```python
from build123d import *

# Parameters (mm, degrees)
BOSS_EXTRUDE1_DEPTH = 18
SKETCH2_R           = 1.5
SKETCH2_W           = 30
SKETCH2_H           = 2.78
CUT_EXTRUDE1_DEPTH  = 7.5
SKETCH3_W           = 3.1
SKETCH3_H           = 6.15
CUT_EXTRUDE2_DEPTH  = 7.5
SKETCH4_W           = 3
SKETCH4_H           = 7.645
CUT_EXTRUDE3_DEPTH  = 5.5
SKETCH5_W           = 6.5
SKETCH5_H           = 2.5
CUT_EXTRUDE4_DEPTH  = 30


with BuildPart() as part:
    # Sketch1 → Boss-Extrude1 (new body, symmetric)
    with BuildSketch(Plane(origin=(0, 0, 0), x_dir=(0, 0, -1), z_dir=(1, 0, 0))):
        Polygon((0, 0), (0, 40.35), (-2, 40.35), (-2, 9.45), (-6.5, 2.78), (-2, 2.78), (-2, 0), align=None)
    extrude(amount=BOSS_EXTRUDE1_DEPTH, both=True)

    # Sketch2 → Cut-Extrude1 (cut, through all)
    with BuildSketch(Plane(origin=(0, 0, 0), x_dir=(-1, 0, 0), z_dir=(0, 0, -1))):
        with Locations((0, 37.1)):
            Circle(SKETCH2_R)
        with Locations((0, 1.39)):
            Rectangle(SKETCH2_W, SKETCH2_H)
    extrude(amount=-CUT_EXTRUDE1_DEPTH, mode=Mode.SUBTRACT)

    # Sketch3 → Cut-Extrude2 (cut, through all)
    with BuildSketch(Plane(origin=(0, 0, 0), x_dir=(-1, 0, 0), z_dir=(0, 0, -1))):
        with Locations((-16.45, 13.5)):
            Rectangle(SKETCH3_W, SKETCH3_H)
        with Locations((16.45, 13.5)):
            Rectangle(SKETCH3_W, SKETCH3_H)
    extrude(amount=-CUT_EXTRUDE2_DEPTH, mode=Mode.SUBTRACT)

    # Sketch4 → Cut-Extrude3 (cut, through all)
    with BuildSketch(Plane.XY.offset(2)):
        with Locations((-16.5, 6.6025)):
            Rectangle(SKETCH4_W, SKETCH4_H)
        with Locations((16.5, 6.6025)):
            Rectangle(SKETCH4_W, SKETCH4_H)
    extrude(amount=CUT_EXTRUDE3_DEPTH, mode=Mode.SUBTRACT)

    # Sketch5 → Cut-Extrude4 (cut)
    with BuildSketch(Plane.ZY.offset(15)):
        with Locations((3.25, 4.03)):
            Rectangle(SKETCH5_W, SKETCH5_H)
    extrude(amount=-CUT_EXTRUDE4_DEPTH, mode=Mode.SUBTRACT)


solid = part.part
```
For this review, take the finished solid that the model builds, in its own axes (mm). A direction names the side the tool comes from. Round coordinates to 2 decimals unless told otherwise and drop trailing zeros. Write each loop counter-clockwise with the first axis right and the second up, starting at its lowest first coordinate (ties: lowest second). Pieces come first, ordered by that corner, then holes. Notation, with made-up numbers: M 24.5,84.5 L 81.5,84.5 A15 ccw 81.5,104.5 Z; hole C 71.25,51 d3. An arc over 180 degrees is marked long. One line per item, written item: value. Start each with the question number.
(1) The part is to be moulded in two halves that separate along Y. For faces 6 (the flat face through (17, 0, 1)), 7 (the flat face through (18, 5, 1)), 8 (the flat face through (-16, 10.425, 1)), say which applies: released by +Y, released by -Y, zero draft, split by the parting line, or undercut.
(2) We need section B-B (x = 0). Give the boundary of the cut face in (y, z).
(3) Machinability: for faces 1 (the flat face through (-15, 7, 3)), 2 (the flat face through (15, 7, 3)), 3 (the flat face through (0, 5.28, 2)), 4 (the flat face through (-16, 16.575, 1)), 5 (the flat face through (14.9, 13, 1)), which of the approach directions +Z, -Z, +X, -X, +Y, -Y give a long, thin tool a straight path to every point of the face, cutting with its end or side? Answer none if there is none.
(4) Insertion check: pin 1 (4 mm diameter, centred on x = 11, y = 23, fed in from +Z); pin 2 (1 mm diameter, centred on y = 13.5, z = 1, fed in from +X); pin 3 (1.4 mm diameter, centred on x = -6, z = 3, fed in from -Y). Each pin has a flat end and moves straight along its axis. Give the tip position at first contact, or say it passes through.
(5) We need section D-D (y = 26). Give the boundary of the cut face in (x, z).
(6) We need section C-C (z = 0.45). Give the boundary of the cut face in (x, y) (3 decimals).
(7) Wall thickness on line 1 (Y direction, x = 0, z = 0.7); line 2 (Z direction, x = -15, y = 26.5); line 3 (Y direction, x = 11, z = 1.15): over which ranges is each line inside the solid? List them lowest first.
(8) We need section A-A (y = 37.1). Give the boundary of the cut face in (x, z), and give its area (3 significant figures).
Result:
1. face 6: released by -Y
1. face 7: zero draft
1. face 8: undercut
2. outline: M 5.28,0 L 35.6,0 L 35.6,2 L 9.45,2 L 5.28,4.81 Z; M 38.6,0 L 40.35,0 L 40.35,2 L 38.6,2 Z
3. face 1: +Z, -X, +Y, -Y
3. face 2: +Z, +X, +Y, -Y
3. face 3: +Z, -Z, -Y
3. face 4: +Z, -Z, -X
3. face 5: +Z, -Z, +X
4. pin 1: z = 2
4. pin 2: x = 14.9
4. pin 3: y = 5.28
5. outline: M -18,0 L 18,0 L 18,2 L -18,2 Z
6. outline: M -18,0 L -15,0 L -15,5.28 L 15,5.28 L 15,0 L 18,0 L 18,10.425 L 14.9,10.425 L 14.9,16.575 L 18,16.575 L 18,40.35 L -18,40.35 L -18,16.575 L -14.9,16.575 L -14.9,10.425 L -18,10.425 Z; hole C 0,37.1 d3
7. line 1: 5.28 to 35.6, 38.6 to 40.35
7. line 2: 0 to 2
7. line 3: 5.28 to 40.35
8. outline: M -18,0 L -1.5,0 L -1.5,2 L -18,2 Z; M 1.5,0 L 18,0 L 18,2 L 1.5,2 Z
8. area: 66.0 mm²
